Autodesk Inventor part; units mm, degrees
ref_plane "YZ Plane" through (0, 0, 0) normal (1, 0, 0) x (0, 1, 0)
ref_plane "XZ Plane" through (0, 0, 0) normal (0, 1, 0) x (-1, 0, 0)
ref_plane "XY Plane" through (0, 0, 0) normal (0, 0, 1) x (1, 0, 0)
sketch "Sketch1" plane through (0, 0, 0) normal (0, 1, 0) x (-1, 0, 0)
  line L0 (0, 0) -> (169, 0)
  line L1 (169, 0) -> (169, -20)
  line L2 (169, -20) -> (0, -20)
  line L3 (0, -20) -> (0, 0)
  dimension "d0" = 169
  dimension "d1" = 20
extrude "Extrusion1" add sketch "Sketch1" along normal blind 2
sketch "Sketch2" plane through (0, 0, 0) normal (0, -1, 0) x (1, 0, 0)
  line L0 (0, 0) -> (0, -20)
  line L1 (0, -10) -> (-169, -10) construction
  line L2 (-169, -20) -> (-169, 0)
  line L3 (-84.5, -10) -> (-84.5, 52.7002) construction
  point P0 (-161.5, -10)
  point P1 (-7.5, -10)
  dimension "d6" = 154
hole "Hole1" at (-161.5, 0, -10) at (-7.5, 0, -10) direction (0, 1, 0) diameter 4 end through all
sketch "Sketch3" plane through (0, 0, 0) normal (0, -1, 0) x (1, 0, 0)
  line L0 (-169, -20) -> (-169, 0) construction
  line L1 (-169, -10) -> (0, -10) construction
  line L2 (0, 0) -> (0, -20) construction
  line L3 (-169, 0.75) -> (0, 0.75)
  line L4 (-169, 0.75) -> (-169, -10)
  line L5 (0, 0.75) -> (0, -10)
  line L6 (-169, -20.75) -> (0, -20.75)
  line L7 (-169, -20.75) -> (-169, -10)
  line L8 (0, -20.75) -> (0, -10)
  dimension "d15" = 21.5
extrude "Extrusion2" cut sketch "Sketch3" against normal blind 10 keep common part
properties part number "ballastBar" material "Steel"
The model under review builds one solid part; all positions refer to its coordinate system, in mm. Give positions to 0.01 mm unless a question says otherwise; leave off trailing zeros. Write each loop counter-clockwise with the first axis right and the second up, starting at its lowest first coordinate (ties: lowest second). Pieces come first, ordered by that corner, then holes. Notation, with made-up numbers: M -26.5,-30 L 28.5,-30 A15 ccw 28.5,-3 Z; hole C -13,18 d6. An arc over 180 degrees is marked long. Answer in a Markdown table with one row per item.
Item 1: Add section A-A on x = -161.5. Give the boundary of the cut face in (y, z), plus the area to 3 significant figures.
Check sheet entries:
| item | result |
|---|---|
| outline | M 0,-20 L 2,-20 L 2,-12 L 0,-12 Z; M 0,-8 L 2,-8 L 2,0 L 0,0 Z |
| area | 32.0 mm2 |
Item 2: For line 1 along X through (y, z) = (0.55, -10); line 2 along Z through (x, y) = (-7.5, 1.2); line 3 along X through (y, z) = (0.35, -8.5), list the stretches that pass through material, from the lowest coordinate up.
Check sheet entries:
| item | result |
|---|---|
| line 1 | -169 to -163.5, -159.5 to -9.5, -5.5 to 0 |
| line 2 | -20 to -12, -8 to 0 |
| line 3 | -169 to -162.82, -160.18 to -8.82, -6.18 to 0 |
Item 3: Add section B-B on z = -10. Give the boundary of the cut face in (x, y).
Check sheet entries:
| item | result |
|---|---|
| outline | M -169,0 L -163.5,0 L -163.5,2 L -169,2 Z; M -159.5,0 L -9.5,0 L -9.5,2 L -159.5,2 Z; M -5.5,0 L 0,0 L 0,2 L -5.5,2 Z |
Item 4: Draft analysis for pull direction X (two halves, no side actions). For faces 1 (the face through (-83, 2, -10)), 2 (the face through (-159.726, 1.014, -10.923)), state which applies: +X half, -X half, draft (parallel to the pull), parting line (faces both ways), or undercut.
Check sheet entries:
| item | result |
|---|---|
| face 1 | draft |
| face 2 | undercut |
